Verification items for the finished model (mm, model axes). A direction names the side the tool comes from. Coordinates: 2 decimals unless noted, no trailing zeros. Order: outer loops, then holes, each group sorted by start corner. A loop starts at its lowest first (then second) coordinate and runs counter-clockwise, first axis right, second up. Notation, with made-up numbers: M 28,14.25 L 58,14.25 A6 ccw 58,21.25 Z; hole C 12,72.5 d4. An arc over 180 degrees is marked long. Write item = value, one per line.
```python
from build123d import *

# Parameters (mm, degrees)
F1_W      = 21
F1_H      = 4
F2_DEPTH  = 17.5
F3_R      = 1.75
F4_DEPTH  = 4.001
F5_W      = 21
F5_H      = 1
F6_DEPTH  = 4
F7_R      = 0.5
F8_DEPTH  = 4
F9_W      = 7
F9_H      = 6.82205
F10_DEPTH = 4


with BuildPart() as f2:
    # F1 (on Top) → F2 (new body)
    with BuildSketch(Plane.XY):
        Rectangle(F1_W, F1_H)
    extrude(amount=F2_DEPTH)

    # F3 (on face) → F4 (cut, through all)
    with BuildSketch(Plane.XZ.offset(2)):
        with Locations((-6, 14.5)):
            Circle(F3_R)
        with Locations((6, 14.5)):
            Circle(F3_R)
        with Locations((6, 2.5)):
            Circle(F3_R)
        with Locations((-6, 2.5)):
            Circle(F3_R)
    extrude(amount=-F4_DEPTH, mode=Mode.SUBTRACT)

    # F5 (on offset) → F6 (cut, symmetric)
    with BuildSketch(Plane.XY.offset(8.5)):
        with Locations((0, 1.5)):
            Rectangle(F5_W, F5_H)
    extrude(amount=F6_DEPTH, both=True, mode=Mode.SUBTRACT)

    # F7 (on offset) → F8 (join, symmetric)
    with BuildSketch(Plane.XY.offset(8.5)):
        with Locations((10, 1)):
            Circle(F7_R)
        with Locations((8, 1)):
            Circle(F7_R)
        with Locations((6, 1)):
            Circle(F7_R)
        with Locations((4, 1)):
            Circle(F7_R)
        with Locations((2, 1)):
            Circle(F7_R)
        with Locations((0, 1)):
            Circle(F7_R)
        with Locations((-2, 1)):
            Circle(F7_R)
        with Locations((-4, 1)):
            Circle(F7_R)
        with Locations((-6, 1)):
            Circle(F7_R)
        with Locations((-8, 1)):
            Circle(F7_R)
        with Locations((-10, 1)):
            Circle(F7_R)
    extrude(amount=F8_DEPTH, both=True)

    # F9 (on offset) → F10 (cut, symmetric)
    with BuildSketch(Plane.XY.offset(8.5)):
        Rectangle(F9_W, F9_H)
    extrude(amount=F10_DEPTH, both=True, mode=Mode.SUBTRACT)


solid = f2.part
```
Item 1: Gauge pin test, flat ends, axial feed: pin 1 (0.8 mm diameter, centred on x = -5, z = 9, fed in from +Y); pin 2 (1 mm diameter, centred on x = 2, z = 11.5, fed in from -Y). Record the tip position at first contact, or that the pin passes through.
Report:
pin_1 = 1
pin_2 = through
Item 2: Release check for a two-part mould opening along Z. For faces 1 (the flat face through (0, 2, 15)), 2 (the flat face through (0, 0, 0)), 3 (the flat face through (3.5, -1, 9)) record: pulls with the +Z half, pulls with the -Z half, needs draft (parallel to the pull), parting line crosses it, or undercut.
Report:
face_1 = needs draft
face_2 = pulls with the -Z half
face_3 = undercut
Item 3: Tool access check on faces 4 (the flat face through (7, 1, 9)), 5 (the flat face through (-3.5, -1, 9)), 6 (the flat face through (0, 2, 2)). Record the directions out of +Z, -Z, +X, -X, +Y, -Y that give a thin tool (end or side, any length) a straight path to the whole face; none if there is none.
Report:
face_4 = +Y
face_5 = +Y, -Y
face_6 = +Z, -Z, +X, -X, +Y
Item 4: Sectioned sample at B-B, the plane x = -6. Enter the section's corners in (y, z), then the cut area to 3 significant figures.
Report:
outline = M -2,0 L 2,0 L 2,0.75 L -2,0.75 Z; M -2,4.25 L 2,4.25 L 2,4.5 L 1.5,4.5 L 1.5,12.5 L 2,12.5 L 2,12.75 L -2,12.75 Z; M -2,16.25 L 2,16.25 L 2,17.5 L -2,17.5 Z
area = 38.0 mm^2
Item 5: Sectioned sample at A-A, the plane z = 11.75. Enter the section's corners in (x, y).
Report:
outline = M -10.5,-2 L -3.5,-2 L -3.5,1 A0.5 ccw -4.5,1 L -5.5,1 A0.5 ccw -6.5,1 L -7.5,1 A0.5 ccw -8.5,1 L -9.5,1 A0.5 ccw -10.5,1 Z; M 3.5,-2 L 10.5,-2 L 10.5,1 A0.5 ccw 9.5,1 L 8.5,1 A0.5 ccw 7.5,1 L 6.5,1 A0.5 ccw 5.5,1 L 4.5,1 A0.5 ccw 3.5,1 Z
Item 6: Scan lines: L1, parallel to Z at x = -1, y = 0.4; L2, parallel to X at y = -1.2, z = 2.75; L3, parallel to Z at x = -6, y = -0.4. Record each from-to range of solid material in increasing order. Write a range as from..to.
Report:
L1 = 0..4.5, 12.5..17.5
L2 = -10.5..-7.73, -4.27..4.27, 7.73..10.5
L3 = 0..0.75, 4.25..12.75, 16.25..17.5
Item 7: Sectioned sample at D-D, the plane x = -1.75. Enter the section's corners in (y, z), then the cut area to 3 significant figures.
Report:
outline = M -2,0 L 2,0 L 2,4.5 L -2,4.5 Z; M -2,12.5 L 2,12.5 L 2,17.5 L -2,17.5 Z
area = 38.0 mm^2
Item 8: Sectioned sample at C-C, the plane y = -1.3. Enter the section's corners in (x, z).
Report:
outline = M -10.5,0 L 10.5,0 L 10.5,17.5 L -10.5,17.5 Z; hole C -6,2.5 d3.5; hole C -6,14.5 d3.5; hole M -3.5,4.5 L 3.5,4.5 L 3.5,12.5 L -3.5,12.5 Z; hole C 6,2.5 d3.5; hole C 6,14.5 d3.5
